The figure shows three views and two pictorial views of one solid part (mm, origin at its lowest corner). Answer the questions. A direction names the side the tool comes from. Coordinates: 2 decimals unless noted, no trailing zeros. Order: outer loops, then holes, each group sorted by start corner. A loop starts at its lowest first (then second) coordinate and runs counter-clockwise, first axis right, second up. Notation, with made-up numbers: (62.25, 82.5) - (81.25, 82.5) arc R33 ccw to (81.25, 111.5) - close; hole circle Ø6 at (-14.75, 30). An arc over 180 degrees is marked (long way). Use one line per item in the form item = value.
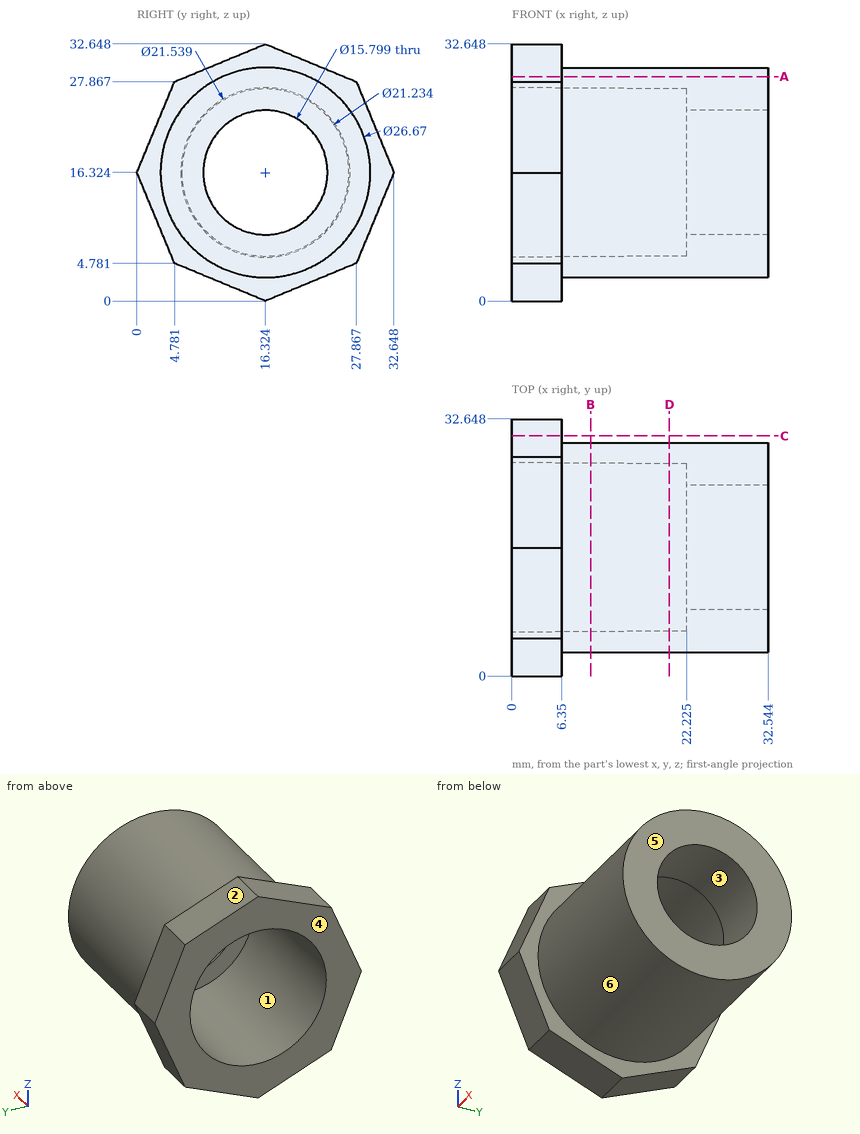
(1) Section D-D, the plane x = 20 is taken. Write down the section's boundary in (y, z) (1 decimal).
Answer list:
outline = circle Ø26.7 at (16.3, 16.3); hole circle Ø21.3 at (16.3, 16.3)
(2) The mould has two halves that part along Z. Classify the marked faces 1, 2, 3 and 4: +Z half, -Z half, draft (parallel to the pull), parting line (faces both ways), or undercut.
Answer list:
face_1 = undercut
face_2 = +Z half
face_3 = undercut
face_4 = draft
(3) Straight lines are drawn through the part: L1, parallel to X at y = 24, z = 21 (1 decimal); L2, parallel to Z at x = 22, y = 14 (1 decimal); L3, parallel to X at y = 13.5, z = 3. For each, find the intervals that lie inside material, in ascending order.
Answer list:
L1 = 22.2 to 32.5
L2 = 3.2 to 6, 26.7 to 29.5
L3 = 0 to 6.35
(4) Section B-B, the plane x = 10 is taken. Write down the section's boundary in (y, z) (1 decimal).
Answer list:
outline = circle Ø26.7 at (16.3, 16.3); hole circle Ø21.4 at (16.3, 16.3)
(5) Which of the six approach directions +Z, -Z, +X, -X, +Y, -Y give full straight-line access (tool end or side, diameter ignored) to the marked faces 5 and 6?
Answer list:
face_5 = +Z, -Z, +X, +Y, -Y
face_6 = +X
(6) Given pin 1 Ø8 at (x, z) = (25.5, 22.5) entering from +Y; pin 2 Ø8 at (x, z) = (21, 11) entering from -Y (1 decimal); pin 3 Ø3 at (x, z) = (10, 28) entering from +Y, each flat-ended and moving along its own axis, determine where each tip first touches the part or whether it passes through.
Answer list:
pin_1 = 29.48
pin_2 = 3.1
pin_3 = 24.94
(7) Section A-A, the plane z = 28.5 is taken. Write down the section's boundary in (x, y), then the cut area to 3 significant figures.
Answer list:
outline = (0, 6.31) - (6.35, 6.31) - (6.35, 10.89) - (32.54, 10.89) - (32.54, 21.76) - (6.35, 21.76) - (6.35, 26.34) - (0, 26.34) - close
area = 412 mm2
(8) Section C-C, the plane y = 30.5 is taken. Write down the section's boundary in (x, z).
Answer list:
outline = (0, 11.14) - (6.35, 11.14) - (6.35, 21.51) - (0, 21.51) - close
